Autodesk Inventor part; units mm, degrees
ref_plane "YZ Plane" through (0, 0, 0) normal (1, 0, 0) x (0, 1, 0)
ref_plane "XZ Plane" through (0, 0, 0) normal (0, 1, 0) x (-1, 0, 0)
ref_plane "XY Plane" through (0, 0, 0) normal (0, 0, 1) x (1, 0, 0)
sketch "Sketch1" plane through (0, 0, 0) normal (0, 1, 0) x (-1, 0, 0)
  line L0 (0, 6.35) -> (-15, 6.35)
  line L1 (-15, 6.35) -> (-15, 2.35)
  line L2 (-15, 2.35) -> (-25, 2.35)
  line L3 (-25, 2.35) -> (-25, -6.35)
  line L4 (-25, -6.35) -> (0, -6.35)
  line L5 (0, -6.35) -> (0, 6.35)
  point P0 (0, 0)
  point P1 (0, 0)
  dimension "d0" = 30
  dimension "d1" = 10
  dimension "d2" = 12.7
  dimension "d3" = 4
revolve "Revolution1" add sketch "Sketch1" angle 360 about axis through (0, 0, -6.35) along (0, 0, 1)
hole "Hole1" at (0, 0, 6.35) direction (0, 0, -1) diameter 7.798 end through all
sketch "Sketch3" plane through (0, 0, -6.35) normal (0, 0, -1) x (-1, 0, 0)
  line L0 (-6.9148, 6.9148) -> (6.9148, 6.9148)
  line L1 (6.9148, 6.9148) -> (6.9148, -6.9148)
  line L2 (6.9148, -6.9148) -> (-6.9148, -6.9148)
  line L3 (-6.9148, -6.9148) -> (-6.9148, 6.9148)
  line L4 (-6.9148, 6.9148) -> (6.9148, -6.9148) construction
  line L5 (6.9148, 6.9148) -> (-6.9148, -6.9148) construction
  point P0 (0, 0)
  dimension "d14" = 19.558
hole "Hole2" at (-6.9148, 6.9148, -6.35) at (-6.9148, -6.9148, -6.35) at (6.9148, -6.9148, -6.35) at (6.9148, 6.9148, -6.35) direction (0, 0, 1) diameter 2.642 end through all
properties part number "Ground_Tracker_TripodMount" material "UHMW, White"
The listing builds one solid part. Answer for the finished solid, in the listing's coordinates (mm). Round coordinates to 2 decimals unless told otherwise and drop trailing zeros. Write each loop counter-clockwise with the first axis right and the second up, starting at its lowest first coordinate (ties: lowest second). Pieces come first, ordered by that corner, then holes. Notation, with made-up numbers: M 85,58.5 L 144,58.5 A31 ccw 144,91.5 Z; hole C 25,29.5 d8. An arc over 180 degrees is marked long. Write each question's results on one line, items separated by ' | '. Start each with the question number.
Item 1: For a pull along Y with two mould halves and no side action, classify faces 1 (the face through (7.421, 8.135, 0.089)), 2 (the face through (-14.985, -0.66, 4.322)), 3 (the face through (11, -11, 2.35)) as pulls with the +Y half, pulls with the -Y half, needs draft (parallel to the pull), parting line crosses it, or undercut.
Item 2: A cutting plane is placed at C-C on y = -7. Write down the section's boundary in (x, z).
Item 3: A cutting plane is placed at A-A on x = 0. Write down the section's boundary in (y, z).
Item 4: A cutting plane is placed at D-D on z = -2.25. Write down the section's boundary in (x, y).
Item 5: Flat-ended cylindrical pins translate along their axes: pin 1 Ø1 at (y, z) = (19.5, -1.5) entering from +X; pin 2 Ø1 at (x, y) = (-5, 17.5) entering from +Z; pin 3 Ø1.6 at (x, y) = (-6.91, -6.91) entering from +Z; pin 4 Ø4 at (y, z) = (-6, -4.5) entering from +X. Find the tip coordinate at first contact, or state that the pin passes through.
Item 6: Straight lines are drawn through the part: L1, parallel to Z at x = 15.5, y = 0; L2, parallel to Y at x = -6.5, z = -2; L3, parallel to Y at x = 6, z = -4.25. For each, find the intervals that lie inside material, in ascending order. Write a range as [from, to].
Check sheet entries:
1) face 1: undercut | face 2: parting line crosses it | face 3: needs draft
2) outline: M -24,-6.35 L -8.23,-6.35 L -8.23,6.35 L -13.27,6.35 L -13.27,2.35 L -24,2.35 Z; M -5.6,-6.35 L 5.6,-6.35 L 5.6,6.35 L -5.6,6.35 Z; M 8.23,-6.35 L 24,-6.35 L 24,2.35 L 13.27,2.35 L 13.27,6.35 L 8.23,6.35 Z
3) outline: M -25,-6.35 L -3.9,-6.35 L -3.9,6.35 L -15,6.35 L -15,2.35 L -25,2.35 Z; M 3.9,-6.35 L 25,-6.35 L 25,2.35 L 15,2.35 L 15,6.35 L 3.9,6.35 Z
4) outline: C 0,0 d50; hole C -6.91,-6.91 d2.64; hole C -6.91,6.91 d2.64; hole C 0,0 d7.8; hole C 6.91,-6.91 d2.64; hole C 6.91,6.91 d2.64
5) pin 1: x = 16.25 | pin 2: z = 2.35 | pin 3: through | pin 4: x = 24.68
6) L1: [-6.35, 2.35] | L2: [-24.14, -8.17], [-5.66, 5.66], [8.17, 24.14] | L3: [-24.27, -7.87], [-5.96, 5.96], [7.87, 24.27]
